Input: part model. Units: mm. Frame: model coordinates. Round coordinates to 2 decimals unless told otherwise and drop trailing zeros. Loops run counter-clockwise (first coordinate to the right, second up) from the corner with the lowest first, then second, coordinate; pieces in that order, holes last. Notation, with made-up numbers: M 50,20.5 L 83,20.5 A24 ccw 83,39.5 Z; hole C 41,84 d9. An arc over 180 degrees is marked long. Return JSON: item names as keys, results as strings. Group by question number.
1) Section B-B (x = 2897). Output: boundary loops of the cut face in (y, z).
2) Contact query for flat-ended pins moving along their axis: P1, Ø2, axis at x = 2794.5, z = 1, coming from the -Y side; P2, Ø2.5, axis at x = 2729.19, y = 1856.63, coming from the +Z side; P3, Ø3, axis at x = 2750, z = 2, coming from the -Y side; P4, Ø2.5, axis at y = 1793, z = 2.5, coming from the -X side. Output: stop coordinate, or through.
3) Section D-D (y = 1773.5). Output: boundary loops of the cut face in (x, z), plus the area to 3 significant figures.
4) Section A-A (y = 1875). Output: boundary loops of the cut face in (x, z).
5) Material intervals for line 1 (Y direction, x = 2695, z = 1.85); line 2 (X direction, y = 1710.5, z = 4.4); line 3 (X direction, y = 1820.5, z = 1.3), sorted ascending. Write a range as from..to.
6) Section C-C (x = 2810). Output: boundary loops of the cut face in (y, z), plus the area to 3 significant figures.
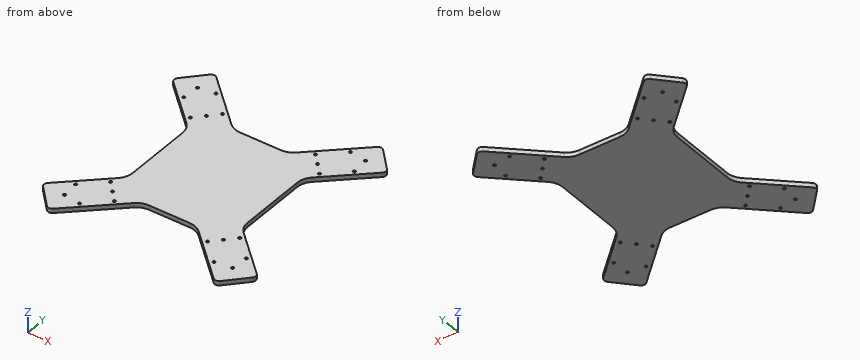
from build123d import *

# Parameters (mm, degrees)
EXTRUDE_1_DEPTH     = 5
SKETCH_3_R          = 1.5
CUT_EXTRUDE_1_DEPTH = 10
SKETCH_4_R          = 1.5
CUT_EXTRUDE_2_DEPTH = 10
SKETCH_5_R          = 1.5
CUT_EXTRUDE_3_DEPTH = 33


with BuildPart() as part:
    # 草图2 → 凸台-拉伸1 (new body)
    with BuildSketch(Plane.XY):
        with BuildLine():
            Line((2769.066394733, 1854.135920645), (2815.285788336, 1854.135920645))
            ThreePointArc((2815.285788336, 1854.135920645), (2822.615812871, 1855.527569285), (2828.925755538, 1859.508846613))
            Line((2828.925755538, 1859.508846613), (2883.306876366, 1910.220062186))
            ThreePointArc((2883.306876366, 1910.220062186), (2886.89136565, 1911.560247813), (2890.373636674, 1909.973285478))
            Line((2890.373636674, 1909.973285478), (2910.833587476, 1888.03267443))
            ThreePointArc((2910.833587476, 1888.03267443), (2912.173773103, 1884.448185146), (2910.586810768, 1880.965914121))
            Line((2910.586810768, 1880.965914121), (2863.536124333, 1837.090439207))
            ThreePointArc((2863.536124333, 1837.090439207), (2858.834890047, 1830.438346554), (2857.176091534, 1822.463365175))
            Line((2857.176091534, 1822.463365175), (2857.176091534, 1745.808476115))
            ThreePointArc((2857.176091534, 1745.808476115), (2858.834890047, 1737.833494737), (2863.536124333, 1731.181402083))
            Line((2863.536124333, 1731.181402083), (2910.586810768, 1687.305927169))
            ThreePointArc((2910.586810768, 1687.305927169), (2912.173773103, 1683.823656144), (2910.833587476, 1680.239166861))
            Line((2910.833587476, 1680.239166861), (2890.373636674, 1658.298555812))
            ThreePointArc((2890.373636674, 1658.298555812), (2886.89136565, 1656.711593477), (2883.306876366, 1658.051779104))
            Line((2883.306876366, 1658.051779104), (2828.925755538, 1708.762994677))
            ThreePointArc((2828.925755538, 1708.762994677), (2822.615812871, 1712.744272005), (2815.285788336, 1714.135920645))
            Line((2815.285788336, 1714.135920645), (2769.066394733, 1714.135920645))
            ThreePointArc((2769.066394733, 1714.135920645), (2761.736370198, 1712.744272005), (2755.426427531, 1708.762994677))
            Line((2755.426427531, 1708.762994677), (2701.045306703, 1658.051779104))
            ThreePointArc((2701.045306703, 1658.051779104), (2697.460817419, 1656.711593477), (2693.978546395, 1658.298555812))
            Line((2693.978546395, 1658.298555812), (2673.518595593, 1680.239166861))
            ThreePointArc((2673.518595593, 1680.239166861), (2672.178409966, 1683.823656144), (2673.765372301, 1687.305927169))
            Line((2673.765372301, 1687.305927169), (2720.816058736, 1731.181402083))
            ThreePointArc((2720.816058736, 1731.181402083), (2725.517293022, 1737.833494737), (2727.176091534, 1745.808476115))
            Line((2727.176091534, 1745.808476115), (2727.176091534, 1822.463365175))
            ThreePointArc((2727.176091534, 1822.463365175), (2725.517293022, 1830.438346554), (2720.816058736, 1837.090439207))
            Line((2720.816058736, 1837.090439207), (2673.765372301, 1880.965914121))
            ThreePointArc((2673.765372301, 1880.965914121), (2672.178409966, 1884.448185146), (2673.518595593, 1888.03267443))
            Line((2673.518595593, 1888.03267443), (2693.978546395, 1909.973285478))
            ThreePointArc((2693.978546395, 1909.973285478), (2697.460817419, 1911.560247813), (2701.045306703, 1910.220062186))
            Line((2701.045306703, 1910.220062186), (2755.426427531, 1859.508846613))
            ThreePointArc((2755.426427531, 1859.508846613), (2761.736370198, 1855.527569285), (2769.066394733, 1854.135920645))
        make_face()
    extrude(amount=EXTRUDE_1_DEPTH)

    # 草图3 → 切除-拉伸1 (cut)
    with BuildSketch(Plane(origin=(0, 0, 0), x_dir=(-1, 0, 0), z_dir=(0, 0, -1))):
        with Locations((-2868.433025626, 1678.758506614)):
            Circle(SKETCH_3_R)
        with Locations((-2888.892976427, 1700.699117662)):
            Circle(SKETCH_3_R)
        with Locations(Location((-2888.892976427, 1867.572723628, 0), (0, 0, 180))):
            Circle(SKETCH_3_R)
        with Locations((-2868.433025626, 1889.513334676)):
            Circle(SKETCH_3_R)
        with Locations((-2695.459206642, 1867.572723628)):
            Circle(SKETCH_3_R)
        with Locations(Location((-2715.919157443, 1889.513334676, 0), (0, 0, 180))):
            Circle(SKETCH_3_R)
        with Locations((-2715.919157443, 1678.758506614)):
            Circle(SKETCH_3_R)
        with Locations(Location((-2695.459206642, 1700.699117662, 0), (0, 0, 180))):
            Circle(SKETCH_3_R)
    extrude(amount=-CUT_EXTRUDE_1_DEPTH, mode=Mode.SUBTRACT)

    # 草图4 → 切除-拉伸2 (cut)
    with BuildSketch(Plane(origin=(0, 0, 0), x_dir=(-1, 0, 0), z_dir=(0, 0, -1))):
        with Locations((-2887.439245446, 1886.727009473)):
            Circle(SKETCH_4_R)
        with Locations(Location((-2696.912937623, 1886.727009473, 0), (0, 0, 180))):
            Circle(SKETCH_4_R)
        with Locations((-2696.912937623, 1681.544831817)):
            Circle(SKETCH_4_R)
        with Locations(Location((-2887.439245446, 1681.544831817, 0), (0, 0, 180))):
            Circle(SKETCH_4_R)
    extrude(amount=-CUT_EXTRUDE_2_DEPTH, mode=Mode.SUBTRACT)

    # 草图5 → 切除-拉伸3 (cut)
    with BuildSketch(Plane(origin=(0, 0, 0), x_dir=(-1, 0, 0), z_dir=(0, 0, -1))):
        with Locations((-2739.420254686, 1700.673634334)):
            Circle(SKETCH_5_R)
        with Locations(Location((-2718.960303884, 1722.614245382, 0), (0, 0, 180))):
            Circle(SKETCH_5_R)
        with Locations((-2729.190279285, 1711.643939858)):
            Circle(SKETCH_5_R)
        with Locations(Location((-2729.190279285, 1856.627901432, 0), (0, 0, 180))):
            Circle(SKETCH_5_R)
        with Locations((-2718.960303884, 1845.657595908)):
            Circle(SKETCH_5_R)
        with Locations(Location((-2739.420254686, 1867.598206957, 0), (0, 0, 180))):
            Circle(SKETCH_5_R)
        with Locations((-2844.931928383, 1867.598206957)):
            Circle(SKETCH_5_R)
        with Locations(Location((-2865.391879185, 1845.657595908, 0), (0, 0, 180))):
            Circle(SKETCH_5_R)
        with Locations((-2855.161903784, 1856.627901432)):
            Circle(SKETCH_5_R)
        with Locations(Location((-2855.161903784, 1711.643939858, 0), (0, 0, 180))):
            Circle(SKETCH_5_R)
        with Locations((-2865.391879185, 1722.614245382)):
            Circle(SKETCH_5_R)
        with Locations(Location((-2844.931928383, 1700.673634334, 0), (0, 0, 180))):
            Circle(SKETCH_5_R)
    extrude(amount=-CUT_EXTRUDE_3_DEPTH, mode=Mode.SUBTRACT)


solid = part.part
Returned:
{
 "1": {"outline": "M 1665.4,0 L 1699.98,0 L 1699.98,5 L 1665.4,5 Z; M 1868.3,0 L 1902.87,0 L 1902.87,5 L 1868.3,5 Z"},
 "2": {"P1": "stops at y = 1714.14", "P2": "passes through", "P3": "stops at y = 1702.3", "P4": "stops at x = 2727.18"},
 "3": {"outline": "M 2727.18,0 L 2857.18,0 L 2857.18,5 L 2727.18,5 Z", "area": "650 mm^2"},
 "4": {"outline": "M 2680.16,0 L 2738.81,0 L 2738.81,5 L 2680.16,5 Z; M 2845.54,0 L 2904.19,0 L 2904.19,5 L 2845.54,5 Z"},
 "5": {"line 1": "y = 1657.46..1699.27, 1702.13..1707.11, 1861.16..1866.14, 1869..1910.81", "line 2": "x = 2698.64..2728.22, 2730.16..2757.57, 2826.78..2854.19, 2856.13..2885.71", "line 3": "x = 2727.18..2857.18"},
 "6": {"outline": "M 1714.14,0 L 1854.14,0 L 1854.14,5 L 1714.14,5 Z", "area": "700 mm^2"}
}
